Verification items for the finished model (mm, model axes). Give positions to 0.01 mm unless a question says otherwise; leave off trailing zeros. Order: outer loops, then holes, each group sorted by start corner. A loop starts at its lowest first (then second) coordinate and runs counter-clockwise, first axis right, second up. Notation, with made-up numbers: (-4.5, 79) -> (0.5, 79) arc R6 cw to (0.5, 85) -> close; hole circle Ø6 at (42.5, 53.25). An arc over 180 degrees is marked (long way). One line per question, with ' | ' between items. Start each with the question number.
Q1. Section check B-B on z = -1. Record the cut outline in (x, y) (3 decimals), plus the area to 3 significant figures.
Q2. Mould release check, pull along Z, two halves, no side actions. Record for faces 1 (the cylindrical face through (-11.574, 1.565, -24.805)), 2 (the cylindrical face through (-11.71, 1.57, -18.98)), 3 (the flat face through (-6.707, 2, 3)): released by +Z, released by -Z, zero draft, split by the parting line, or undercut.
Q3. Go/stop test with a flat-tipped pin: pin 1 (4 mm diameter, centred on x = -11.47, z = -2.79, fed in from -Y). Record where the tip stops, or that it passes through.
Q4. Section check D-D on y = 1.6. Give the number of separate pieces and of enclosed holes in the cut face, plus the area to 3 significant figures.
Q5. Material ranges on probe 1 along Z at (x, y) = (-11.5, 1.3); probe 2 along Z at (x, y) = (-11, 0.4); probe 3 along Z at (x, y) = (-9.75, 2.35), recorded low to high. Write a range as [from, to].
Q6. Section check A-A on x = -11. Record the cut outline in (y, z) (3 decimals).
Q7. Section check C-C on x = -8.75. Record the cut outline in (y, z) (3 decimals), plus the area to 3 significant figures.
from build123d import *

# Parameters (mm, degrees)
SKETCH2_R           = 1.0922
SKETCH2_R_2         = 3.175
SKETCH2_R_3         = 1.1303
BOSS_EXTRUDE2_DEPTH = 3.175


with BuildPart() as part:
    # Sketch2 → Boss-Extrude2 (new body)
    with BuildSketch(Plane(origin=(0, 0, 0), x_dir=(1, 0, 0), z_dir=(0, 1, 0))):
        with BuildLine():
            Line((-6.706711203, 20.043284588), (-6.706711203, -6.456715412))
            Line((-6.706711203, -6.456715412), (-6.706711203, -26.456715412))
            ThreePointArc((-6.706711203, -26.456715412), (-11.469211203, -31.219215412), (-16.231711203, -26.456715412))
            Line((-16.231711203, -26.456715412), (-16.231711203, -6.456715412))
            Line((-16.231711203, -6.456715412), (-16.231711203, 20.043284588))
            ThreePointArc((-16.231711203, 20.043284588), (-11.469211203, 24.805784588), (-6.706711203, 20.043284588))
        make_face()
        with Locations((-11.469211203, 20.043284588)):
            Circle(SKETCH2_R, mode=Mode.SUBTRACT)
        with Locations((-11.469211203, 2.793284588)):
            Circle(SKETCH2_R_2, mode=Mode.SUBTRACT)
        with Locations((-11.469211203, -26.456715412)):
            Circle(SKETCH2_R_3, mode=Mode.SUBTRACT)
    extrude(amount=BOSS_EXTRUDE2_DEPTH)


solid = part.part
Filled in:
1) outline: (-16.232, 0) -> (-14.089, 0) -> (-14.089, 3.175) -> (-16.232, 3.175) -> close; (-8.849, 0) -> (-6.707, 0) -> (-6.707, 3.175) -> (-8.849, 3.175) -> close | area: 13.6 mm²
2) face 1: released by -Z | face 2: undercut | face 3: zero draft
3) pin 1: through
4) separate pieces: 1 | enclosed holes: 3 | area: 475 mm²
5) probe 1: [-24.81, -21.14], [-18.95, -5.97], [0.38, 25.33], [27.59, 31.22] | probe 2: [-24.78, -21.03], [-19.06, -5.93], [0.35, 25.43], [27.49, 31.2] | probe 3: [-24.48, -5.46], [-0.12, 30.9]
6) outline: (0, -24.783) -> (3.175, -24.783) -> (3.175, -21.03) -> (0, -21.03) -> close; (0, -19.057) -> (3.175, -19.057) -> (3.175, -5.933) -> (0, -5.933) -> close; (0, 0.347) -> (3.175, 0.347) -> (3.175, 25.428) -> (0, 25.428) -> close; (0, 27.485) -> (3.175, 27.485) -> (3.175, 31.196) -> (0, 31.196) -> close
7) outline: (0, -23.953) -> (3.175, -23.953) -> (3.175, -4.432) -> (0, -4.432) -> close; (0, -1.154) -> (3.175, -1.154) -> (3.175, 30.367) -> (0, 30.367) -> close | area: 162 mm²
